The model under review builds one solid part; all positions refer to its coordinate system, in mm. A direction names the side the tool comes from. Give positions to 0.01 mm unless a question says otherwise; leave off trailing zeros. Order: outer loops, then holes, each group sorted by start corner. A loop starts at its lowest first (then second) coordinate and runs counter-clockwise, first axis right, second up. Notation, with made-up numbers: (-32, 64) - (-20, 64) arc R32 ccw to (-20, 96) - close; hole circle Ø8 at (32.25, -10.5). An arc over 180 degrees is marked (long way). Put each result on its own line as item: value.
```python
from build123d import *

# Parameters (mm, degrees)
SKETCH_1_W = 0.7
SKETCH_1_H = 0.05


with BuildPart() as part:
    # 草图1 → 旋转1 (revolve)
    with BuildSketch(Plane.XY):
        Polygon((2.5, 4), (2.5, 0), (3.2, 0), (3.2, 0.3), (5, 0.3), (5, 0), (7, 0), (7, 1), (6, 1), (6, 3.95), (5, 3.95), (5, 3.7), (3.2, 3.7), (3.2, 4), align=None)
        with Locations((2.85, -0.025)):
            Rectangle(SKETCH_1_W, SKETCH_1_H)
        with Locations((2.85, 4.025)):
            Rectangle(SKETCH_1_W, SKETCH_1_H)
    revolve_1 = revolve(axis=Axis((0, -1000, 0), (0, 1, 0)))

    # 镜向1: 旋转1 across plane
    add(revolve_1.mirror(Plane.ZX.offset(4)))


solid = part.part
```
(1) The part is to be moulded in two halves that separate along X. For faces 1 (the flat face through (3.3, 3.7, 1)), 2 (the cylindrical face through (6.466, 7.493, 2.681)), 3 (the cylindrical face through (-2.539, 0.127, 1.947)), 4 (the flat face through (2, -0.05, 2)), say which applies: pulls with the +X half, pulls with the -X half, needs draft (parallel to the pull), parting line crosses it, or undercut.
The answers:
face 1: undercut
face 2: parting line crosses it
face 3: undercut
face 4: needs draft
(2) Clearance check with flat-ended pins moving along their axes: pin 1 Ø3.5 at (x, z) = (2.5, -2.5) entering from -Y; pin 2 Ø4 at (y, z) = (6, -4) entering from +X; pin 3 Ø1.5 at (x, y) = (3, 6) entering from +Z. State where each tip first meets the part, or that it passes through.
The answers:
pin 1: y = -0.05
pin 2: x = 6.62
pin 3: z = 5.56
(3) Take a section at C-C, the plane y = 3. Write out the cut boundary in (x, z), then the cut area to 3 significant figures.
The answers:
outline: circle Ø12 at (0, 0); hole circle Ø5 at (0, 0)
area: 93.5 mm^2
(4) Wall thickness on L1, parallel to X at y = 4.2, z = 0; L2, parallel to X at y = 7.9, z = 0: over which ranges is each line inside the solid? List them lowest first.
The answers:
L1: -6 to -5, -3.2 to -2.5, 2.5 to 3.2, 5 to 6
L2: -7 to -5, -3.2 to -2.5, 2.5 to 3.2, 5 to 7
(5) For faces 5 (the flat face through (-3.3, 0.3, 1)), 6 (the flat face through (2, 8.05, 2)), 7 (the flat face through (6, 1, -2)), 8 (the cylindrical face through (-0.54, 4.06, 2.44)), 9 (the cylindrical face through (4.77, 7.85, -1.5)), list the 3-axis set-ups (+Z, -Z, +X, -X, +Y, -Y) from which the entire face can be reached by the end or side of a thin tool; tool diameter is ignored.
The answers:
face 5: -Y
face 6: +Z, -Z, +X, -X, +Y
face 7: none
face 8: +Y, -Y
face 9: +Y
